```python
from build123d import *

# Parameters (mm, degrees)
F0_W     = 18.2
F0_H     = 8
F1_DEPTH = 2.7
F2_W     = 15
F2_H     = 8
F3_DEPTH = 2
F4_SIZE  = 0.8


with BuildPart() as f1:
    # F0 (on Top) → F1 (new body)
    with BuildSketch(Plane.XY):
        Rectangle(F0_W, F0_H)
    extrude(amount=F1_DEPTH)

    # F2 (on face) → F3 (cut)
    with BuildSketch(Plane.XY.offset(2.7)):
        Rectangle(F2_W, F2_H)
    extrude(amount=-F3_DEPTH, mode=Mode.SUBTRACT)

    # F4
    f4_edges = [f1.edges().sort_by_distance(p)[0] for p in [
        (-9.1, 0, 0),
        (9.1, 0, 0),
    ]]
    chamfer(f4_edges, length=F4_SIZE)


solid = f1.part
```
For this review, take the finished solid that the model builds, in its own axes (mm). A direction names the side the tool comes from. Round coordinates to 2 decimals unless told otherwise and drop trailing zeros. Loops run counter-clockwise (first coordinate to the right, second up) from the corner with the lowest first, then second, coordinate; pieces in that order, holes last.
(1) Tool access review of faces 1 (the flat face through (0, 0, 0.7)), 2 (the flat face through (8, 0, 2.7)): name each direction out of +Z, -Z, +X, -X, +Y, -Y from which nothing blocks a thin tool from reaching the whole face with its end or side.
Returned:
face 1: +Z, +Y, -Y
face 2: +Z, +X, -X, +Y, -Y
(2) Wall thickness on line 1 along X through (y, z) = (1, 2.4); line 2 along Z through (x, y) = (-5.75, -3.5); line 3 along X through (y, z) = (-0.5, 0.45): over which ranges is each line inside the solid? List them lowest first.
Returned:
line 1: x = -9.1 to -7.5, 7.5 to 9.1
line 2: z = 0 to 0.7
line 3: x = -8.75 to 8.75
(3) Clearance check with flat-ended pins moving along their axes: P1, Ø1, axis at x = 5.5, z = 1, coming from the +Y side; P2, Ø4, axis at x = -2, y = 1, coming from the +Z side. State where each tip first meets the part, or that it passes through.
Returned:
P1: stops at y = 4
P2: stops at z = 0.7
(4) Mouldability with a two-part tool opening along X and no side actions: class faces 3 (the flat face through (9.1, 0, 2)), 4 (the flat face through (7.5, 0, 2)), 5 (the flat face through (-8, 0, 2.7)) as released by +X, released by -X, zero draft, split by the parting line, or undercut.
Returned:
face 3: released by +X
face 4: undercut
face 5: zero draft
(5) We need section C-C (x = -4.75). Give the boundary of the cut face in (y, z).
Returned:
outline: (-4, 0) - (4, 0) - (4, 0.7) - (-4, 0.7) - close
(6) We need section A-A (z = 2). Give the boundary of the cut face in (x, y), plus the area to 3 significant figures.
Returned:
outline: (-9.1, -4) - (-7.5, -4) - (-7.5, 4) - (-9.1, 4) - close; (7.5, -4) - (9.1, -4) - (9.1, 4) - (7.5, 4) - close
area: 25.6 mm2
(7) We need section B-B (y = -1). Give the boundary of the cut face in (x, z), plus the area to 3 significant figures.
Returned:
outline: (-9.1, 0.8) - (-8.3, 0) - (8.3, 0) - (9.1, 0.8) - (9.1, 2.7) - (7.5, 2.7) - (7.5, 0.7) - (-7.5, 0.7) - (-7.5, 2.7) - (-9.1, 2.7) - close
area: 18.5 mm2
